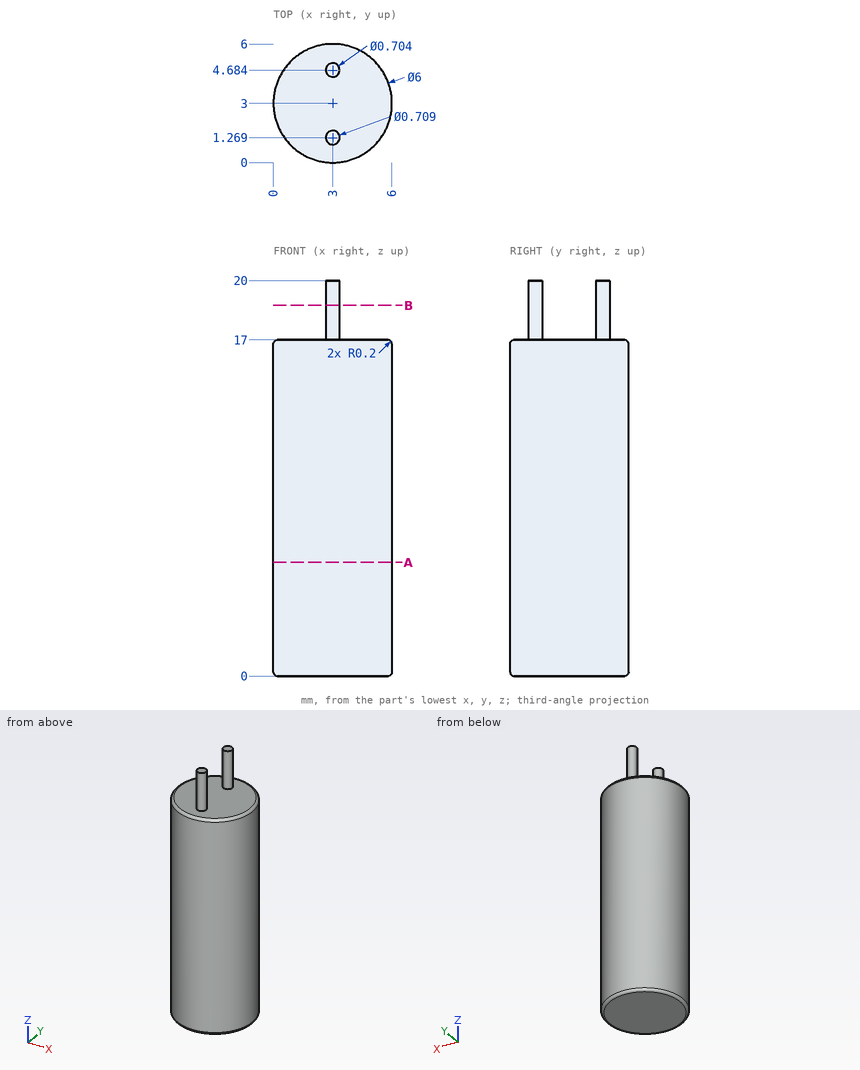
Input: dimensioned drawing with shaded views. Units: mm. Origin: part minimum x, y, z. Give positions to 0.01 mm unless a question says otherwise; leave off trailing zeros. Loops run counter-clockwise (first coordinate to the right, second up) from the corner with the lowest first, then second, coordinate; pieces in that order, holes last. Notation, with made-up numbers: (2.5, 77) -> (24.5, 77) arc R16 ccw to (24.5, 86) -> close; hole circle Ø11 at (19.25, -13). An arc over 180 degrees is marked (long way). Use a Markdown table: item, result. Add a question column.
1) Line query: line 1 along Z through (x, y) = (2, 4.5); line 2 along X through (y, z) = (5.25, 9.75) (1 decimal); line 3 along Y through (x, z) = (4.75, 6) (1 decimal). Output: solid intervals per line, ascending. Write a range as [from, to].
2) First-contact query: pin 1 (2 mm diameter, centred on x = 2.5, y = 3, fed in from +Z); pin 2 (2 mm diameter, centred on x = 5.5, y = 3.5, fed in from -Z); pin 3 (2 mm diameter, centred on x = 1.5, z = 9, fed in from +Y); pin 4 (1 mm diameter, centred on x = 1, z = 16.5, fed in from -Y). Flat tips, straight axial feed; report the tip coordinate or a pass-through.
3) Section query A-A, the plane z = 5.75. Return the cut outline in (x, y).
4) Section query B-B, the plane z = 18.75. Return the cut outline in (x, y) (1 decimal).
Numbers:
| question | item | result |
|---|---|---|
| 1 | line 1 | z = [0, 17] |
| 1 | line 2 | x = [1, 5] |
| 1 | line 3 | y = [0.6, 5.4] |
| 2 | pin 1 | stops at z = 17 |
| 2 | pin 2 | stops at z = 0 |
| 2 | pin 3 | stops at y = 5.96 |
| 2 | pin 4 | stops at y = 0.4 |
| 3 | outline | circle Ø6 at (3, 3) |
| 4 | outline | circle Ø0.7 at (3, 1.3); circle Ø0.7 at (3, 4.7) |
